For this review, take the finished solid that the model builds, in its own axes (mm). A direction names the side the tool comes from. Coordinates: 2 decimals unless noted, no trailing zeros. Write each loop counter-clockwise with the first axis right and the second up, starting at its lowest first coordinate (ties: lowest second). Pieces come first, ordered by that corner, then holes.
```python
from build123d import *

# Parameters (mm, degrees)
SKETCH1_W           = 68.58
SKETCH1_H           = 53.34
BOSS_EXTRUDE1_DEPTH = 2.54
SKETCH2_W           = 3.81
SKETCH2_H           = 3.81
SKETCH2_R           = 1.27
BOSS_EXTRUDE2_DEPTH = 12.7
SKETCH3_W           = 3.81
SKETCH3_H           = 3.81
SKETCH3_R           = 1.27
BOSS_EXTRUDE3_DEPTH = 12.7


with BuildPart() as part:
    # Sketch1 → Boss-Extrude1 (new body)
    with BuildSketch(Plane(origin=(0, 0, 0), x_dir=(1, 0, 0), z_dir=(0, 1, 0))):
        with Locations((34.29, 26.67)):
            Rectangle(SKETCH1_W, SKETCH1_H)
    extrude(amount=BOSS_EXTRUDE1_DEPTH)

    # Sketch2 → Boss-Extrude2 (add)
    with BuildSketch(Plane(origin=(0, 2.54, 0), x_dir=(1, 0, 0), z_dir=(0, 1, 0))):
        with Locations((13.97, 2.54)):
            Rectangle(SKETCH2_W, SKETCH2_H)
        with Locations((13.97, 2.54)):
            Circle(SKETCH2_R, mode=Mode.SUBTRACT)
    extrude(amount=BOSS_EXTRUDE2_DEPTH)

    # Sketch3 → Boss-Extrude3 (add)
    with BuildSketch(Plane(origin=(0, 2.54, 0), x_dir=(1, 0, 0), z_dir=(0, 1, 0))):
        with Locations((15.24, 50.8)):
            Rectangle(SKETCH3_W, SKETCH3_H)
        with Locations((15.24, 50.8)):
            Circle(SKETCH3_R, mode=Mode.SUBTRACT)
        with Locations((66.04, 35.56)):
            Rectangle(SKETCH3_W, SKETCH3_H)
        with Locations((66.04, 35.56)):
            Circle(SKETCH3_R, mode=Mode.SUBTRACT)
        with Locations((66.04, 7.62)):
            Rectangle(SKETCH3_W, SKETCH3_H)
        with Locations((66.04, 7.62)):
            Circle(SKETCH3_R, mode=Mode.SUBTRACT)
    extrude(amount=BOSS_EXTRUDE3_DEPTH)


solid = part.part
```
Q1. Add section A-A (y = 3.75). State the section outline as (x, z) points (3 decimals), then the cut area to 3 significant figures.
Ans:
outline: (12.065, -4.445) - (15.875, -4.445) - (15.875, -0.635) - (12.065, -0.635) - close; (13.335, -52.705) - (17.145, -52.705) - (17.145, -48.895) - (13.335, -48.895) - close; (64.135, -37.465) - (67.945, -37.465) - (67.945, -33.655) - (64.135, -33.655) - close; (64.135, -9.525) - (67.945, -9.525) - (67.945, -5.715) - (64.135, -5.715) - close; hole circle Ø2.54 at (13.97, -2.54); hole circle Ø2.54 at (15.24, -50.8); hole circle Ø2.54 at (66.04, -35.56); hole circle Ø2.54 at (66.04, -7.62)
area: 37.8 mm2
Q2. Add section C-C (z = -35.56). State the section outline as (x, y) points (3 decimals).
Ans:
outline: (0, 0) - (68.58, 0) - (68.58, 2.54) - (67.945, 2.54) - (67.945, 15.24) - (67.31, 15.24) - (67.31, 2.54) - (64.77, 2.54) - (64.77, 15.24) - (64.135, 15.24) - (64.135, 2.54) - (0, 2.54) - close
Q3. Draft analysis for pull direction X (two halves, no side actions). For faces 6 (the flat face through (15, 9, -48.895)), 7 (the flat face through (66, 2.54, -8)), 8 (the flat face through (64.135, 9, -36)), 9 (the flat face through (67.945, 9, -36)), state which applies: +X half, -X half, draft (parallel to the pull), parting line (faces both ways), or undercut.
Ans:
face 6: draft
face 7: undercut
face 8: -X half
face 9: +X half
Q4. Clearance check with flat-ended pins moving along their axes: pin 1 Ø4 at (x, y) = (66, 8.5) entering from -Z (3 decimals); pin 2 Ø3 at (x, y) = (15.5, 12) entering from +Z (3 decimals); pin 3 Ø1.9 at (x, y) = (15.5, 7.5) entering from -Z (3 decimals); pin 4 Ø6 at (x, y) = (45.5, 8.5) entering from +Z. State where each tip first meets the part, or that it passes through.
Ans:
pin 1: stops at z = -37.465
pin 2: stops at z = -0.635
pin 3: stops at z = -52.705
pin 4: passes through
Q5. Tool access review of faces 1 (the flat face through (66, 9, -37.465)), 2 (the flat face through (64.135, 9, -8)), 3 (the flat face through (14, 9, -0.635)), 4 (the cylindrical face through (15.14, 8.8, -2.05)), 5 (the flat face through (66, 9, -9.525)): name each direction out of +Z, -Z, +X, -X, +Y, -Y from which nothing blocks a thin tool from reaching the whole face with its end or side.
Ans:
face 1: -Z, +X, -X, +Y
face 2: +Z, -Z, -X, +Y
face 3: +Z, +X, -X, +Y
face 4: +Y
face 5: +X, -X, +Y
Q6. Add section B-B (x = 66.04). State the section outline as (y, z) points (3 decimals), then the cut area to 3 significant figures.
Ans:
outline: (0, -53.34) - (2.54, -53.34) - (2.54, -37.465) - (15.24, -37.465) - (15.24, -36.83) - (2.54, -36.83) - (2.54, -34.29) - (15.24, -34.29) - (15.24, -33.655) - (2.54, -33.655) - (2.54, -9.525) - (15.24, -9.525) - (15.24, -8.89) - (2.54, -8.89) - (2.54, -6.35) - (15.24, -6.35) - (15.24, -5.715) - (2.54, -5.715) - (2.54, 0) - (0, 0) - close
area: 168 mm2
Q7. Add section D-D (z = -47). State the section outline as (x, y) points.
Ans:
outline: (0, 0) - (68.58, 0) - (68.58, 2.54) - (0, 2.54) - close
Q8. For probe 1 along Z at (x, y) = (66.04, 7) (3 decimals); probe 2 along X at (y, z) = (11, -2.54) (3 decimals); probe 3 along X at (y, z) = (7, -50.8) (3 decimals), list the stretches that pass through material, from the lowest coordinate up.
Ans:
probe 1: z = -37.465 to -36.83, -34.29 to -33.655, -9.525 to -8.89, -6.35 to -5.715
probe 2: x = 12.065 to 12.7, 15.24 to 15.875
probe 3: x = 13.335 to 13.97, 16.51 to 17.145
